from build123d import *

# Parameters (mm, degrees)
F0_R     = 50
F1_DEPTH = 20
F2_R     = 20
F3_DEPTH = 45
F4_W     = 5
F4_H     = 60
F5_DEPTH = 45
F6_R     = 19
F7_DEPTH = 50
F8_W     = 5
F8_H     = 60
F9_DEPTH = 45


with BuildPart() as f1:
    # F0 (on Right) → F1 (new body)
    with BuildSketch(Plane.YZ):
        with Locations((0, 57.614021)):
            Circle(F0_R)
    extrude(amount=F1_DEPTH)

    # F2 (on face) → F3 (join)
    with BuildSketch(Plane(origin=(0, 0, 0), x_dir=(0, -1, 0), z_dir=(-1, 0, 0))):
        with Locations((0, 57.614021)):
            Circle(F2_R)
    extrude(amount=F3_DEPTH)

    # F4 (on Right) → F5 (join)
    with BuildSketch(Plane.YZ):
        with Locations((-22.020652, 40.254378)):
            Rectangle(F4_W, F4_H)
    extrude(amount=-F5_DEPTH)

    # F6 (on face) → F7 (join)
    with BuildSketch(Plane(origin=(-45, 0, 0), x_dir=(0, -1, 0), z_dir=(-1, 0, 0))):
        with Locations((0, 57.614021)):
            Circle(F6_R)
    extrude(amount=F7_DEPTH)

    # F8 (on Right) → F9 (join)
    with BuildSketch(Plane.YZ):
        with Locations((21.119455, 42.110385)):
            Rectangle(F8_W, F8_H)
    extrude(amount=-F9_DEPTH)


solid = f1.part
Work out the finished part from the listing and answer in its coordinate system (mm). A direction names the side the tool comes from. Give positions to 0.01 mm unless a question says otherwise; leave off trailing zeros. Write each loop counter-clockwise with the first axis right and the second up, starting at its lowest first coordinate (ties: lowest second). Pieces come first, ordered by that corner, then holes. Notation, with made-up numbers: M 80.25,0.25 L 125.25,0.25 A20 ccw 125.25,25.25 Z; hole C 60.5,-9 d11. An arc over 180 degrees is marked long. Answer as CSV lines item,"result".
Q1. A cutting plane is placed at C-C on y = 0. Write down the section's boundary in (x, z).
A:
outline,"M -95,38.61 L -45,38.61 L -45,37.61 L 0,37.61 L 0,7.61 L 20,7.61 L 20,107.61 L 0,107.61 L 0,77.61 L -45,77.61 L -45,76.61 L -95,76.61 Z"
Q2. Find the intervals of material crossed by probe 1 along Y at (x, z) = (-37.5, 67); probe 2 along Y at (x, z) = (-1.5, 58); probe 3 along X at (y, z) = (23, 23), in increasing order. Write a range as [from, to].
A:
probe 1,"y = [-24.52, -19.52], [-17.66, 17.66], [18.62, 23.62]"
probe 2,"y = [-24.52, 23.62]"
probe 3,"x = [-45, 20]"
Q3. A cutting plane is placed at B-B on x = -23. Write down the section's boundary in (y, z).
A:
outline,"M -24.52,10.25 L -19.52,10.25 L -19.52,53.26 A20 ccw 18.62,50.31 L 18.62,12.11 L 23.62,12.11 L 23.62,72.11 L 18.62,72.11 L 18.62,64.92 A20 ccw -19.52,61.97 L -19.52,70.25 L -24.52,70.25 Z"
Q4. Given P1, Ø1.5, axis at x = -25, y = -23, coming from the +Z side; P2, Ø2.5, axis at x = -28.5, y = -23, coming from the -Z side; P3, Ø3, axis at x = -39.5, z = 45.5, coming from the -Y side, each flat-ended and moving along its own axis, determine where each tip first touches the part or whether it passes through.
A:
P1,"stops at z = 70.25"
P2,"stops at z = 10.25"
P3,"stops at y = -24.52"
Q5. The mould has two halves that part along Y. Classify faces 6 (the flat face through (-22, 21, 12.11)), 7 (the cylindrical face through (-22.18, -1.19, 37.65)), 8 (the flat face through (-22, -24.521, 40)): +Y half, -Y half, draft (parallel to the pull), parting line (faces both ways), or undercut.
A:
face 6,"draft"
face 7,"undercut"
face 8,"-Y half"
Q6. A cutting plane is placed at A-A on z = 42.5. Write down the section's boundary in (x, y).
A:
outline,"M -95,-11.51 L -45,-11.51 L -45,-13.1 L 0,-13.1 L 0,-19.52 L -45,-19.52 L -45,-24.52 L 0,-24.52 L 0,-47.66 L 20,-47.66 L 20,47.66 L 0,47.66 L 0,23.62 L -45,23.62 L -45,18.62 L 0,18.62 L 0,13.1 L -45,13.1 L -45,11.51 L -95,11.51 Z"
Q7. A cutting plane is placed at D-D on x = -55. Write down the section's boundary in (y, z), plus the area to 3 significant figures.
A:
outline,"C 0,57.61 d38"
area,"1,130 mm²"
Q8. A tool of negligible diameter and unlimited length cuts with its end or side. For faces 1 (the flat face through (-22, -22, 70.254)), 2 (the flat face through (-22, 23.619, 42)), 3 (the flat face through (0, -23, 12)), 4 (the flat face through (-22, 21, 72.11)), 5 (the flat face through (-22, 18.619, 31)), from which of +Z, -Z, +X, -X, +Y, -Y can it reach the whole face along a straight path? Write none if from no direction.
A:
face 1,"+Z, -X, -Y"
face 2,"+Z, -Z, -X, +Y"
face 3,"-Z, +X, -Y"
face 4,"+Z, -X, +Y"
face 5,"-Z, -X"
